Geometry check sheet. Reference: the model listing, model coordinates, mm. Face numbers are marked on the shaded views. A direction names the side the tool comes from. Round coordinates to 2 decimals unless told otherwise and drop trailing zeros. Order: outer loops, then holes, each group sorted by start corner. A loop starts at its lowest first (then second) coordinate and runs counter-clockwise, first axis right, second up.
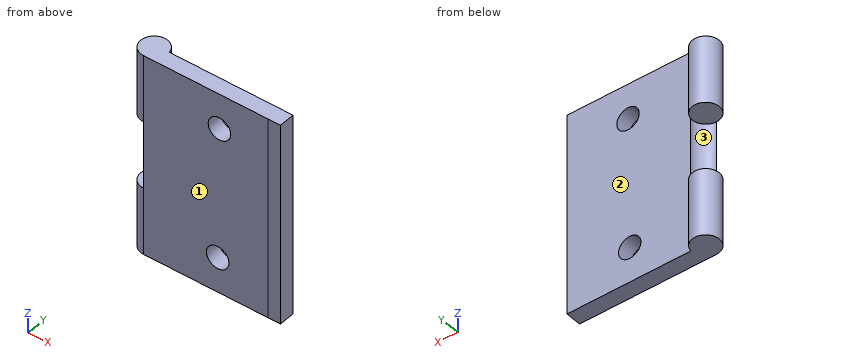
Autodesk Inventor part; units mm, degrees
ref_plane "YZ Plane" through (0, 0, 0) normal (1, 0, 0) x (0, 1, 0)
ref_plane "XZ Plane" through (0, 0, 0) normal (0, 1, 0) x (-1, 0, 0)
ref_plane "XY Plane" through (0, 0, 0) normal (0, 0, 1) x (1, 0, 0)
sketch "Sketch11" plane through (0, 0, 0) normal (0, 0, 1) x (1, 0, 0)
  line L0 (0, 0) -> (27.764, 0)
  line L1 (27.764, 0) -> (27.764, 3.519)
  line L2 (27.764, 3.519) -> (0, 3.519)
  line L3 (0, 3.519) -> (0, 0)
  circle A0 centre (0, 3) radius 3
  point P0 (2.9548, 3.519)
  dimension "d25" = 27.764
  dimension "d26" = 3.519
  dimension "d27" = 6
extrude "Extrusion5" add sketch "Sketch11" along normal blind 45
ref_plane "Work Plane3" through (0, 0, 30) normal (0, 0, 1) x (1, 0, 0)
sketch "Sketch12" plane through (0, 0, 30) normal (0, 0, 1) x (1, 0, 0)
  circle A0 centre (0, 3) radius 3
  point P0 (0, 0)
  dimension "d32" = 6
extrude "Extrusion6" cut sketch "Sketch12" against normal blind 15
sketch "Sketch13" plane through (27.764, 0, 0) normal (1, 0, 0) x (0, 0, -1)
  point P0 (0, 0)
sketch "Sketch14" plane through (2.9548, 3.519, 0) normal (0, 1, 0) x (1, 0, 0)
  line L0 (24.8092, 0) -> (24.8092, -45)
  line L1 (24.8092, 0) -> (30.3097, 0)
  line L2 (30.3097, 0) -> (30.3097, -45)
  line L3 (30.3097, -45) -> (24.8092, -45)
  line L4 (24.8092, -45) -> (24.8092, 0)
  point P0 (-2.9548, 0)
  dimension "d35" = 45
extrude "Extrusion7" add sketch "Sketch14" against normal blind 3.5
sketch "Sketch15" plane through (2.9548, 3.519, 15) normal (0, 1, 0) x (1, 0, 0)
  line L0 (30.3097, 15) -> (30.3097, -30)
  line L1 (24.8092, 15) -> (30.3097, 15)
  line L2 (30.3097, -30) -> (27.5595, -30)
  line L3 (27.5595, -30) -> (27.5595, 15)
  line L4 (27.5595, 15) -> (30.3097, 15)
  line L5 (30.3097, 15) -> (30.3097, -30)
  point P0 (-2.9548, 15)
extrude "Extrusion8" cut sketch "Sketch15" against normal blind 3.5
sketch "Sketch16" plane through (1.0163, 3.519, 45.1466) normal (0, 1, 0) x (1, 0, 0)
  point P0 (-2.9547, 45)
  point P1 (15.912, 7.9951)
  point P2 (15.5243, 37.2981)
hole "Hole2" at (16.9284, 3.519, 37.1515) at (16.5406, 3.519, 7.8485) direction (0, -1, 0) diameter 5 end through all
properties part number "final right" material "Stainless Steel"
(1) Depth check by flat-ended pin: P1, Ø8, axis at x = 16.93, z = 37.15, coming from the +Y side; P2, Ø2, axis at x = 29, z = 14, coming from the -Y side; P3, Ø1, axis at x = 21, y = 4.5, coming from the +Z side. Enter the tip coordinate at first touch or a pass-through.
Returned:
P1: stops at y = 3.52
P2: stops at y = 0.02
P3: passes through
(2) Sectioned sample at C-C, the plane y = 2.4. Record the cut outline in (x, z), and give its area (3 significant figures).
Returned:
outline: (-2.94, 0) - (30.51, 0) - (30.51, 45) - (-2.94, 45) - (-2.94, 30) - (2.94, 30) - (2.94, 15) - (-2.94, 15) - close; hole circle Ø5 at (16.54, 7.85); hole circle Ø5 at (16.93, 37.15)
area: 1,380 mm2
(3) Sectioned sample at A-A, the plane y = 4.85. Record the cut outline in (x, z).
Returned:
outline: (-2.36, 0) - (2.36, 0) - (2.36, 15) - (-2.36, 15) - close; (-2.36, 30) - (2.36, 30) - (2.36, 45) - (-2.36, 45) - close
(4) Set-up check for the marked faces 1, 2 and 3: record each of +Z, -Z, +X, -X, +Y, -Y from which the full face is reachable in a straight line by a thin tool's end or side.
Returned:
face 1: +Z, -Z, +X, -X, -Y
face 2: +Z, -Z, +X, +Y
face 3: -X
(5) Material ranges on line 1 (Z direction, x = -1, y = 2.75); line 2 (Z direction, x = 15, y = 3.35); line 3 (Y direction, x = 26.5, z = 28.5), recorded low to high.
Returned:
line 1: z = 0 to 15, 30 to 45
line 2: z = 0 to 5.88, 9.82 to 35.56, 38.74 to 45
line 3: y = 0 to 3.52
